Input: part model. Units: mm. Frame: model coordinates. Face numbers are marked on the shaded views. A direction names the side the tool comes from. Coordinates: 2 decimals unless noted, no trailing zeros. Order: outer loops, then holes, each group sorted by start corner. A loop starts at its lowest first (then second) coordinate and runs counter-clockwise, first axis right, second up.
from build123d import *

# Parameters (mm, degrees)
SKETCH002_R  = 14.7
PAD002_DEPTH = 40
SKETCH003_W  = 1
SKETCH003_H  = 40
POCKET_DEPTH = 30
FILLET_R     = 3


with BuildPart() as part:
    # Sketch002 (on Binder) → Pad002 (new body)
    with BuildSketch(Plane(origin=(0, 0, -5), x_dir=(1, 0, 0), z_dir=(0, 0, -1))):
        Circle(SKETCH002_R)
    extrude(amount=-PAD002_DEPTH)

    # Sketch003 (on Face3 of Pad002) → Pocket (cut)
    with BuildSketch(Plane.XY.offset(35)):
        Rectangle(SKETCH003_W, SKETCH003_H)
    extrude(amount=-POCKET_DEPTH, mode=Mode.SUBTRACT)

    # Fillet
    fillet_edges = [part.edges().sort_by_distance(p)[0] for p in [
        (-14.7, 0, 35),
        (-0.5, 0, 35),
        (10.569768, -10.216164, 35),
        (0.5, 0, 35),
        (10.569768, 10.216164, 35),
    ]]
    fillet(fillet_edges, radius=FILLET_R)


solid = part.part
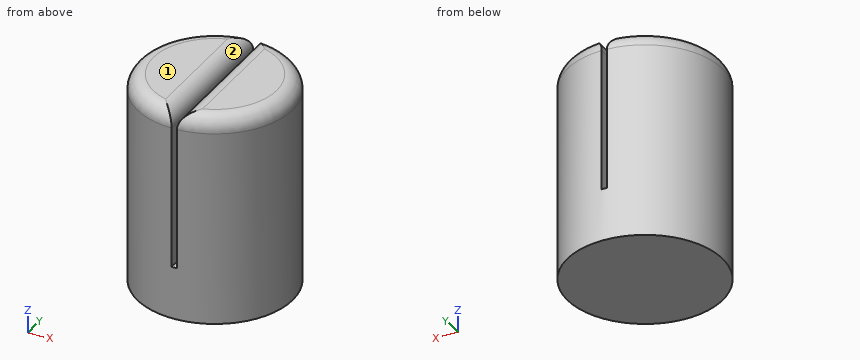
Item 1: Cut plane B-B on z = 31.5. Return loops of the section in (x, y), then the cut area to 3 significant figures.
Response values:
outline: (-0.5, -14.69) - (-0.5, 14.69) arc R14.7 ccw to start; (0.5, -14.69) arc R14.7 ccw to (0.5, 14.69) - close
area: 649 mm2
Item 2: Pin query (flat end, axial travel): pin 1 Ø3 at (y, z) = (8.5, 17) entering from +X; pin 2 Ø5 at (x, z) = (1.5, 29.5) entering from -Y; pin 3 Ø12 at (x, z) = (10, 9) entering from -Y. Return the tip coordinate at first contact, or that it passes through.
Response values:
pin 1: stops at x = 12.93
pin 2: stops at y = -14.69
pin 3: stops at y = -14.15
Item 3: Ray query, probe 1 along X at (y, z) = (5, 15); probe 2 along X at (y, z) = (-5.5, 17); probe 3 along Y at (x, z) = (6, 5). Return the intervals inside material, ascending.
Response values:
probe 1: x = -13.82 to -0.5, 0.5 to 13.82
probe 2: x = -13.63 to -0.5, 0.5 to 13.63
probe 3: y = -13.42 to 13.42
Item 4: Access query for the marked faces 1 and 2. Directions: +Z, -Z, +X, -X, +Y, -Y. A direction counts if a zero-diameter tool reaches every point of the face in a straight line with its end or side. Return the directions, or none.
Response values:
face 1: +Z, +X, -X, +Y, -Y
face 2: +Z, +Y, -Y
Item 5: Cut plane C-C on x = 0. Return loops of the section in (y, z).
Response values:
outline: (-14.7, -5) - (14.7, -5) - (14.7, 5) - (-14.7, 5) - close
Item 6: Cut plane A-A on y = 0. Return loops of the section in (x, z), then the cut area to 3 significant figures.
Response values:
outline: (-14.7, -5) - (14.7, -5) - (14.7, 32) arc R3 ccw to (11.7, 35) - (3.5, 35) arc R3 ccw to (0.5, 32) - (0.5, 5) - (-0.5, 5) - (-0.5, 32) arc R3 ccw to (-3.5, 35) - (-11.7, 35) arc R3 ccw to (-14.7, 32) - close
area: 1,140 mm2
